from build123d import *

# Parameters (mm, degrees)
F0_R         = 48.5
F0_R_2       = 30.5
F1_DEPTH     = 9
F2_R         = 37.75
F2_R_2       = 30.5
F3_DEPTH     = 35
F4_R         = 5
F5_R         = 1.25
F5_R_2       = 1.255
F6_DEPTH     = 30
F7_T4_ANGLE  = 359.64
F7_S5_R      = 37.75
F7_T6_DEPTH  = 9
F7_T10_ANGLE = 359.64
F7_S11_R     = 37.75
F7_T12_DEPTH = 9
F7_T16_ANGLE = 359.64
F7_S17_R     = 37.75
F7_T18_DEPTH = 9
F7_T22_ANGLE = 359.64
F7_S23_R     = 37.75
F7_T24_DEPTH = 9
F8_SIZE      = 2
F9_SIZE      = 3


# Not quite as in the source:
# - a fillet or chamfer that OpenCascade refuses, or shapes differently, is made with other operations: its cross-section is extruded or revolved along the edge and cut away or added


with BuildPart() as f1:
    # F0 (on Top) → F1 (new body)
    with BuildSketch(Plane.XY):
        Circle(F0_R)
        Circle(F0_R_2, mode=Mode.SUBTRACT)
    extrude(amount=F1_DEPTH)

    # F2 (on face) → F3 (join)
    with BuildSketch(Plane.XY.offset(9)):
        Circle(F2_R)
        Circle(F2_R_2, mode=Mode.SUBTRACT)
    extrude(amount=F3_DEPTH)

    # F4
    f4_edges = [f1.edges().sort_by_distance(p)[0] for p in [
        (-37.75, 0, 44),
    ]]
    fillet(f4_edges, radius=F4_R)

    # F5 (on face) → F6 (join)
    with BuildSketch(Plane.XY.offset(9)):
        with Locations((0, 37.75)):
            Circle(F5_R)
        with Locations((-37.75, 0)):
            Circle(F5_R_2)
        with Locations((0, -37.75)):
            Circle(F5_R_2)
        with Locations((37.75, 0)):
            Circle(F5_R_2)
    extrude(amount=F6_DEPTH)

    # F7: chamfer of 1.249 x 15 on 4 edges, made by hand


with BuildPart() as f7_tool2:
    # F7_s3 → F7_t4 (revolve)
    with BuildSketch(Plane(origin=(-0.0003725763, 0.1185943423, 0), x_dir=(0, 0, 1), z_dir=(0.0031415875, -0.9999950652, 0))):
        Polygon((24, 36.4948137114), (39, 37.7438137114), (39, 36.4948137114), align=None)
    revolve(axis=Axis((-37.75, 0, 39), (0, 0, 1)), revolution_arc=F7_T4_ANGLE)

    # F7_s5 → F7_t6 (cut, symmetric)
    with BuildSketch(Plane.XY.offset(31.5)):
        Circle(F7_S5_R)
    extrude(amount=F7_T6_DEPTH, both=True, mode=Mode.SUBTRACT)


with BuildPart() as f1_1:
    add(f1.part)

    # F7_t1: cut F7_tool2
    add(f7_tool2.part, mode=Mode.SUBTRACT)


with BuildPart() as f7_tool8:
    # F7_s9 → F7_t10 (revolve)
    with BuildSketch(Plane(origin=(0.1185943423, 0.0003725763, 0), x_dir=(0, 0, 1), z_dir=(-0.9999950652, -0.0031415875, 0))):
        Polygon((24, 36.4998137114), (39, 37.7488137114), (39, 36.4998137114), align=None)
    revolve(axis=Axis((0, 37.75, 39), (0, 0, 1)), revolution_arc=F7_T10_ANGLE)

    # F7_s11 → F7_t12 (cut, symmetric)
    with BuildSketch(Plane.XY.offset(31.5)):
        Circle(F7_S11_R)
    extrude(amount=F7_T12_DEPTH, both=True, mode=Mode.SUBTRACT)


with BuildPart() as f1_2:
    add(f1_1.part)

    # F7_t7: cut F7_tool8
    add(f7_tool8.part, mode=Mode.SUBTRACT)


with BuildPart() as f7_tool14:
    # F7_s15 → F7_t16 (revolve)
    with BuildSketch(Plane(origin=(-0.1185943423, -0.0003725763, 0), x_dir=(0, 0, 1), z_dir=(0.9999950652, 0.0031415875, 0))):
        Polygon((24, 36.4948137114), (39, 37.7438137114), (39, 36.4948137114), align=None)
    revolve(axis=Axis((0, -37.75, 39), (0, 0, 1)), revolution_arc=F7_T16_ANGLE)

    # F7_s17 → F7_t18 (cut, symmetric)
    with BuildSketch(Plane.XY.offset(31.5)):
        Circle(F7_S17_R)
    extrude(amount=F7_T18_DEPTH, both=True, mode=Mode.SUBTRACT)


with BuildPart() as f1_3:
    add(f1_2.part)

    # F7_t13: cut F7_tool14
    add(f7_tool14.part, mode=Mode.SUBTRACT)


with BuildPart() as f7_tool20:
    # F7_s21 → F7_t22 (revolve)
    with BuildSketch(Plane(origin=(0.0003725763, -0.1185943423, 0), x_dir=(0, 0, 1), z_dir=(-0.0031415875, 0.9999950652, 0))):
        Polygon((24, 36.4948137114), (39, 37.7438137114), (39, 36.4948137114), align=None)
    revolve(axis=Axis((37.75, 0, 39), (0, 0, 1)), revolution_arc=F7_T22_ANGLE)

    # F7_s23 → F7_t24 (cut, symmetric)
    with BuildSketch(Plane.XY.offset(31.5)):
        Circle(F7_S23_R)
    extrude(amount=F7_T24_DEPTH, both=True, mode=Mode.SUBTRACT)


with BuildPart() as f1_4:
    add(f1_3.part)

    # F7_t19: cut F7_tool20
    add(f7_tool20.part, mode=Mode.SUBTRACT)

    # F8
    f8_edges = [f1_4.edges().sort_by_distance(p)[0] for p in [
        (-30.5, 0, 0),
    ]]
    chamfer(f8_edges, length=F8_SIZE)

    # F9
    f9_edges = [f1_4.edges().sort_by_distance(p)[0] for p in [
        (-48.5, 0, 9),
    ]]
    chamfer(f9_edges, length=F9_SIZE)


solid = f1_4.part
Design review of the part built by this model. Coordinates are the model's own, in mm. A direction names the side the tool comes from. Give positions to 0.01 mm unless a question says otherwise; leave off trailing zeros. Order: outer loops, then holes, each group sorted by start corner. A loop starts at its lowest first (then second) coordinate and runs counter-clockwise, first axis right, second up.
1. For pin 1 Ø6 at (x, z) = (-27.5, 31.5) entering from +Y; pin 2 Ø6 at (x, z) = (21, 5.5) entering from +Y; pin 3 Ø1 at (x, z) = (32, 21) entering from +Y, all flat-tipped, find the tip position at first contact; note any pin that passes through.
Solution:
pin 1: stops at y = 28.72
pin 2: stops at y = 45.04
pin 3: stops at y = 20.8
2. Mouldability with a two-part tool opening along Y and no side actions: class faces 1 (the cylindrical face through (-26.396, 26.987, 23.79)), 2 (the cylindrical face through (26.398, -26.985, 23.79)), 3 (the conical face through (-6.64, -29.9, 1.87)), 4 (the cylindrical face through (39.005, -0.028, 16.395)) as +Y half, -Y half, draft (parallel to the pull), parting line (faces both ways), or undercut.
Solution:
face 1: +Y half
face 2: -Y half
face 3: undercut
face 4: parting line
3. To check wall thickness, follow L1, parallel to Y at x = 9.5, z = 34; L2, parallel to Y at x = 0, z = 26; L3, parallel to X at y = 8, z = 5. State the ranges of each line that lie inside material, in increasing order.
Solution:
L1: y = -36.54 to -28.98, 28.98 to 36.54
L2: y = -38.84 to -30.5, 30.5 to 38.83
L3: x = -47.84 to -29.43, 29.43 to 47.84
4. Add section B-B, the plane z = 37.5. State the section outline as (x, y) points.
Solution:
outline: (-37.75, -0.13) arc R37.75 ccw to (-0.13, -37.75) arc R0.13 ccw to (0.13, -37.75) arc R37.75 ccw to (37.75, -0.13) arc R0.13 ccw to (37.75, 0.13) arc R37.75 ccw to (0.13, 37.75) arc R0.13 ccw to (-0.13, 37.75) arc R37.75 ccw to (-37.75, 0.13) arc R0.13 ccw to start; hole circle Ø61 at (0, 0)
5. Tool access review of faces 5 (the cylindrical face through (26.983, 26.4, 23.79)), 6 (the cylindrical face through (-26.985, -26.398, 23.79)), 7 (the flat face through (-17, 34, 9)): name each direction out of +Z, -Z, +X, -X, +Y, -Y from which nothing blocks a thin tool from reaching the whole face with its end or side.
Solution:
face 5: +Z, +X, +Y
face 6: +Z, -X, -Y
face 7: +Z
6. Add section A-A, the plane z = 22. State the section outline as (x, y) points (3 decimals).
Solution:
outline: (-37.729, -1.255) arc R37.75 ccw to (-1.255, -37.729) arc R1.255 ccw (long way) to (1.255, -37.729) arc R37.75 ccw to (37.729, -1.255) arc R1.255 ccw (long way) to (37.729, 1.255) arc R37.75 ccw to (1.25, 37.729) arc R1.25 ccw (long way) to (-1.25, 37.729) arc R37.75 ccw to (-37.729, 1.255) arc R1.255 ccw (long way) to start; hole circle Ø61 at (0, 0)
